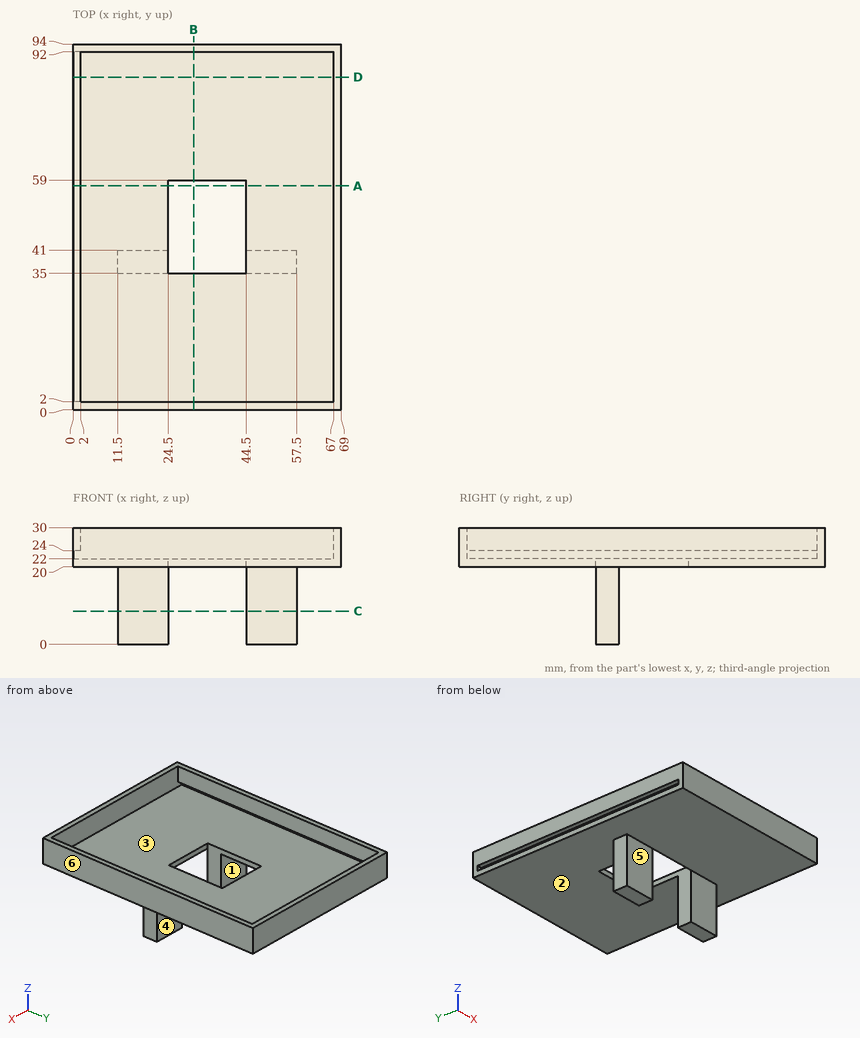
Design review of the part shown in the three views and the two pictorial views. Dimensions are in mm from the part's minimum x, y and z. A direction names the side the tool comes from. Round coordinates to 2 decimals unless told otherwise and drop trailing zeros. Write each loop counter-clockwise with the first axis right and the second up, starting at its lowest first coordinate (ties: lowest second). Pieces come first, ordered by that corner, then holes.
Item 1: Wall thickness on L1, parallel to Y at x = 18, z = 26.25; L2, parallel to X at y = 54.5, z = 21.5; L3, parallel to X at y = 75, z = 28.5: over which ranges is each line inside the solid? List them lowest first.
Item 2: Consider section A-A on y = 57.5. Give the boundary of the cut face in (x, z), and give its area (3 significant figures).
Item 3: For pin 1 Ø1.5 at (x, y) = (45.5, 12.5) entering from -Z; pin 2 Ø3 at (y, z) = (37.5, 14.5) entering from -X; pin 3 Ø1.8 at (y, z) = (39.5, 14.5) entering from +X, all flat-tipped, find the tip position at first contact; note any pin that passes through.
Item 4: Consider section C-C on z = 8.5. Give the boundary of the cut face in (x, y).
Item 5: Consider section B-B on x = 31. Give the boundary of the cut face in (y, z).
Item 6: For the marked faces 4, 5 and 6, list the 3-axis set-ups (+Z, -Z, +X, -X, +Y, -Y) from which the entire face can be reached by the end or side of a thin tool; tool diameter is ignored.
Item 7: Draft analysis for pull direction Y (two halves, no side actions). For the marked faces 1, 2 and 3, state which applies: released by +Y, released by -Y, zero draft, split by the parting line, or undercut.
Item 8: Consider section D-D on y = 85.5. Give the boundary of the cut face in (x, z), and give its area (3 significant figures).
Check values:
1. L1: y = 0 to 2, 92 to 94
1. L2: x = 0 to 24.5, 44.5 to 69
1. L3: x = 0 to 2, 67 to 69
2. outline: (0, 20) - (24.5, 20) - (24.5, 22) - (0, 22) - close; (0, 24) - (2, 24) - (2, 30) - (0, 30) - close; (44.5, 20) - (69, 20) - (69, 30) - (67, 30) - (67, 22) - (44.5, 22) - close
2. area: 126 mm2
3. pin 1: stops at z = 20
3. pin 2: stops at x = 11.5
3. pin 3: stops at x = 57.5
4. outline: (11.5, 35) - (24.5, 35) - (24.5, 41) - (11.5, 41) - close; (44.5, 35) - (57.5, 35) - (57.5, 41) - (44.5, 41) - close
5. outline: (0, 20) - (35, 20) - (35, 22) - (2, 22) - (2, 30) - (0, 30) - close; (59, 20) - (94, 20) - (94, 30) - (92, 30) - (92, 22) - (59, 22) - close
6. face 4: -Z, +X, -X, +Y
6. face 5: -Z, +X, -X, -Y
6. face 6: +Z, -Z, +X, +Y, -Y
7. face 1: released by +Y
7. face 2: zero draft
7. face 3: undercut
8. outline: (0, 20) - (69, 20) - (69, 30) - (67, 30) - (67, 22) - (0, 22) - close; (0, 24) - (2, 24) - (2, 30) - (0, 30) - close
8. area: 166 mm2
